```python
from build123d import *

# Parameters (mm, degrees)
SKETCH1_W                                      = 57.14999999999999
SKETCH1_H                                      = 43.17999999999999
BASE_DEPTH                                     = 57.15
POCKET_DEPTH                                   = 47.9552
LINACTHOLE_DEPTH                               = 68.44465304974146
ROLLMOTORHOLE_REACH                            = 85.656
DVIHOLE_REACH                                  = 69.445
CBORE_FOR_4_SOCKET_HEAD_CAP_SCREW1_D           = 3.2639
CBORE_FOR_4_SOCKET_HEAD_CAP_SCREW1_CBORE_D     = 6.35
CBORE_FOR_4_SOCKET_HEAD_CAP_SCREW1_CBORE_DEPTH = 2.8448
CBORE_FOR_8_SOCKET_HEAD_CAP_SCREW1_D           = 4.4958
CBORE_FOR_8_SOCKET_HEAD_CAP_SCREW1_CBORE_D     = 7.9375
CBORE_FOR_8_SOCKET_HEAD_CAP_SCREW1_CBORE_DEPTH = 4.1656
FILLET1_R                                      = 0.254


with BuildPart() as part:
    # Sketch1 → Base (new body)
    with BuildSketch(Plane(origin=(0, 0, 0), x_dir=(1, 0, 0), z_dir=(0, 1, 0))):
        Rectangle(SKETCH1_W, SKETCH1_H)
    extrude(amount=BASE_DEPTH)

    # Sketch2 → Pocket (cut)
    with BuildSketch(Plane(origin=(0, 57.15, 0), x_dir=(1, 0, 0), z_dir=(0, 1, 0))):
        Polygon((26.035000000000004, -19.05), (-26.03499999999999, -19.050000000000008), (-26.03499999999999, 19.049999999999994), (26.035000000000004, 19.050000000000004), align=None)
    extrude(amount=-POCKET_DEPTH, mode=Mode.SUBTRACT)

    # Sketch3 → LinActHole (cut, through all)
    with BuildSketch(Plane(origin=(0, 0, 0), x_dir=(-1, 0, 0), z_dir=(0, -1, 0))):
        Polygon((7.492999999999988, -7.7470000000000026), (-10.79500000000001, -7.747000000000003), (-10.79500000000001, 7.746999999999995), (7.492999999999988, 7.746999999999996), align=None)
    extrude(amount=-LINACTHOLE_DEPTH, mode=Mode.SUBTRACT)

    # Sketch4 → RollMotorHole (cut, up to next)
    with BuildSketch(Plane.ZY.offset(28.575), mode=Mode.PRIVATE) as rollmotorhole_sk1:
        Polygon((15.747999999999998, 57.15), (-4.317999999999999, 57.150000000000006), (-4.317999999999998, 47.625), (15.747999999999998, 47.625000000000014), align=None)
    rollmotorhole_tool1 = extrude(rollmotorhole_sk1.sketch, amount=-ROLLMOTORHOLE_REACH, mode=Mode.PRIVATE) & part.part
    add(rollmotorhole_tool1.solids().sort_by_distance((-28.575, 52.3875, 5.715))[0], mode=Mode.SUBTRACT)

    # Sketch5 → DviHole (cut, up to next)
    with BuildSketch(Plane.XZ, mode=Mode.PRIVATE) as dvihole_sk1:
        with BuildLine():
            Line((17.624947542752004, -13.715999999999998), (24.228947542752003, -13.716))
            Line((24.228947542752003, -13.716), (24.228947542752003, 13.716000000000003))
            Line((24.228947542752003, 13.716000000000003), (17.624947542752004, 13.716000000000005))
            ThreePointArc((17.624947542752004, 13.716000000000005), (15.828896318538174, 12.972051224213832), (15.084947542752005, 11.176000000000002))
            Line((15.084947542752005, 11.176000000000002), (15.084947542752005, -11.175999999999998))
            ThreePointArc((15.084947542752005, -11.175999999999998), (15.828896318538174, -12.972051224213828), (17.624947542752004, -13.715999999999998))
        make_face()
    dvihole_tool1 = extrude(dvihole_sk1.sketch, amount=-DVIHOLE_REACH, mode=Mode.PRIVATE) & part.part
    add(dvihole_tool1.solids().sort_by_distance((19.701649, 0, 0))[0], mode=Mode.SUBTRACT)

    # CBORE for #4 Socket Head Cap Screw1 (through all)
    with Locations(Plane(origin=(0, 0, 0), x_dir=(-1, 0, 0), z_dir=(0, -1, 0))):
        with Locations((-19.656947543, 16.256), (-19.656947543, -16.256)):
            CounterBoreHole(CBORE_FOR_4_SOCKET_HEAD_CAP_SCREW1_D / 2, CBORE_FOR_4_SOCKET_HEAD_CAP_SCREW1_CBORE_D / 2, CBORE_FOR_4_SOCKET_HEAD_CAP_SCREW1_CBORE_DEPTH)

    # CBORE for #8 Socket Head Cap Screw1 (through all)
    with Locations(Plane(origin=(0, 0, 0), x_dir=(-1, 0, 0), z_dir=(0, -1, 0))):
        with Locations((3.175, 14.605), (3.175, -14.605)):
            CounterBoreHole(CBORE_FOR_8_SOCKET_HEAD_CAP_SCREW1_D / 2, CBORE_FOR_8_SOCKET_HEAD_CAP_SCREW1_CBORE_D / 2, CBORE_FOR_8_SOCKET_HEAD_CAP_SCREW1_CBORE_DEPTH)

    # Fillet1
    # the kernel refuses this fillet: 0.254 mm, written as the material it takes off along each edge
    with BuildSketch(Plane(origin=(21.56194754300001, 2.8448, 13.716000000000006), x_dir=(1, 0, -5.46e-15), z_dir=(0, -1, 0))) as fillet1_piece_1:
        with BuildLine():
            CenterArc((0.6508256982823206, 0.25399999999999956), FILLET1_R, 138.18968510422349, 131.8103148957768)
            ThreePointArc((0.4615052761873327, 0.4233333333333256), (0.24121576475939824, 0.20026008045803986), (0, 0))
            Line((0, 0), (0.650825698282322, 0))
        make_face()
    extrude(amount=4.471864245705805, mode=Mode.SUBTRACT)
    with BuildSketch(Plane(origin=(17.751947542999993, 2.8448, 13.716000000000006), x_dir=(-0.9977003347705025, 0, -0.06777936263220105), z_dir=(0, -1, 0))) as fillet1_piece_2:
        with BuildLine():
            CenterArc((0.5964633639844708, -0.2525550871245977), FILLET1_R, 96.11431340709308, 122.7684855876463)
            Line((0.3987417282209075, -0.4119983521155698), (0.37896956464454973, -0.4279426786146676))
            ThreePointArc((0.37896956464454973, -0.4279426786146676), (0.19043822259418336, -0.21464439732501625), (-0.01658222975058737, -0.01924031331602186))
            Line((-0.01658222975058737, -0.01924031331602186), (0.00172159581085787, 0.02534158850317019))
            ThreePointArc((0.00172159581085787, 0.02534158850317019), (0.12842953857413036, 0.01673360943207212), (0.5667037799709318, 0.02525550871246005))
            Line((0.5667037799709318, 0.02525550871246005), (0.5694091966994345, 0))
        make_face()
    extrude(amount=4.278191101484826, mode=Mode.SUBTRACT)
    with BuildSketch(Plane(origin=(17.751947543000007, 2.8448, -13.715999999999996), x_dir=(-0.9977003347705027, 0, 0.06777936263219668), z_dir=(0, -1, 0))) as fillet1_piece_3:
        with BuildLine():
            CenterArc((0.5964633639844823, 0.25255508712459757), FILLET1_R, 141.1172010052604, 122.76848558764627)
            Line((0.3987417282209198, 0.4119983521155705), (0.37896956464456205, 0.4279426786146684))
            ThreePointArc((0.37896956464456205, 0.4279426786146684), (0.19043822259419124, 0.21464439732501767), (-0.01658222975058728, 0.01924031331602193))
            Line((-0.01658222975058728, 0.01924031331602193), (0.00172159581085776, -0.02534158850317019))
            ThreePointArc((0.00172159581085776, -0.02534158850317019), (0.12842953857414433, -0.01673360943206995), (0.5667037799709422, -0.02525550871246003))
            Line((0.5667037799709422, -0.02525550871246003), (0.5694091966994449, 0))
        make_face()
    extrude(amount=4.278191101484849, mode=Mode.SUBTRACT)
    with BuildSketch(Plane(origin=(21.561947542999995, 2.8448, -13.715999999999996), x_dir=(1, 0, -5.46e-15), z_dir=(0, -1, 0))) as fillet1_piece_4:
        with BuildLine():
            CenterArc((0.6508256982823268, -0.25399999999999956), FILLET1_R, 90.0000000000003, 131.81031489577913)
            ThreePointArc((0.46150527618734805, -0.42333333333333484), (0.2412157647594075, -0.20026008045804258), (0, 0))
            Line((0, 0), (0.6508256982823255, 0))
        make_face()
    extrude(amount=4.471864245705815, mode=Mode.SUBTRACT)


solid = part.part
```
Design review of the part built by this model. Coordinates are the model's own, in mm. A direction names the side the tool comes from. Round coordinates to 2 decimals unless told otherwise and drop trailing zeros. Write each loop counter-clockwise with the first axis right and the second up, starting at its lowest first coordinate (ties: lowest second). Pieces come first, ordered by that corner, then holes. Notation, with made-up numbers: (3.25, 19.25) -> (16.25, 19.25) arc R8 cw to (16.25, 30.25) -> close; hole circle Ø7 at (39.25, -40). An arc over 180 degrees is marked (long way). Answer in a Markdown table with one row per item.
Q1. Draft analysis for pull direction Z (two halves, no side actions). For faces 5 (the face through (-11, 9.195, 0)), 6 (the face through (0, 0, -10)), state which applies: +Z half, -Z half, draft (parallel to the pull), parting line (faces both ways), or undercut.
The answers:
| item | result |
|---|---|
| face 5 | undercut |
| face 6 | draft |
Q2. Take a section at B-B, the plane x = 8. State the section outline as (y, z) points, then the cut area to 3 significant figures.
The answers:
| item | result |
|---|---|
| outline | (0, -21.59) -> (57.15, -21.59) -> (57.15, -19.05) -> (9.19, -19.05) -> (9.19, -7.75) -> (0, -7.75) -> close; (0, 7.75) -> (9.19, 7.75) -> (9.19, 19.05) -> (57.15, 19.05) -> (57.15, 21.59) -> (0, 21.59) -> close |
| area | 498 mm² |
Q3. Take a section at C-C, the plane y = 44. State the section outline as (x, z) points (3 decimals).
The answers:
| item | result |
|---|---|
| outline | (-28.575, -21.59) -> (28.575, -21.59) -> (28.575, 21.59) -> (-28.575, 21.59) -> close; hole (-26.035, -19.05) -> (26.035, -19.05) -> (26.035, 19.05) -> (-26.035, 19.05) -> close |
Q4. Clearance check with flat-ended pins moving along their axes: pin 1 Ø7 at (x, z) = (-3.175, -14.605) entering from -Y; pin 2 Ø6 at (x, z) = (-3.175, 14.605) entering from +Y; pin 3 Ø0.8 at (x, z) = (-27.5, 5.5) entering from +Y (3 decimals). State where each tip first meets the part, or that it passes through.
The answers:
| item | result |
|---|---|
| pin 1 | y = 4.17 |
| pin 2 | y = 9.19 |
| pin 3 | y = 47.625 |
Q5. For faces 1 (the face through (-5, 4.166, -13)), 2 (the face through (-27, 52, -4.318)), 3 (the face through (0, 34, -19.05)), 4 (the face through (15.849, 4.533, 12.992)), list the 3-axis set-ups (+Z, -Z, +X, -X, +Y, -Y) from which the entire face can be reached by the end or side of a thin tool; tool diameter is ignored.
The answers:
| item | result |
|---|---|
| face 1 | -Y |
| face 2 | -X, +Y |
| face 3 | +Y |
| face 4 | +Y, -Y |
Q6. Take a section at A-A, the plane z = -0.5. State the section outline as (x, y) points (3 decimals).
The answers:
| item | result |
|---|---|
| outline | (-28.575, 0) -> (-7.493, 0) -> (-7.493, 9.195) -> (-26.035, 9.195) -> (-26.035, 47.625) -> (-28.575, 47.625) -> close; (10.795, 0) -> (15.085, 0) -> (15.085, 9.195) -> (10.795, 9.195) -> close; (24.229, 0) -> (28.575, 0) -> (28.575, 57.15) -> (26.035, 57.15) -> (26.035, 9.195) -> (24.229, 9.195) -> close |
Q7. Take a section at D-D, the plane y = 5.5. State the section outline as (x, z) points (3 decimals), then the cut area to 3 significant figures.
The answers:
| item | result |
|---|---|
| outline | (-28.575, -21.59) -> (28.575, -21.59) -> (28.575, 21.59) -> (-28.575, 21.59) -> close; hole (-7.493, -7.747) -> (10.795, -7.747) -> (10.795, 7.747) -> (-7.493, 7.747) -> close; hole circle Ø4.496 at (-3.175, -14.605); hole circle Ø4.496 at (-3.175, 14.605); hole (15.085, -11.176) arc R2.54 ccw to (17.625, -13.716) -> (24.229, -13.716) -> (24.229, 13.716) -> (17.625, 13.716) arc R2.54 ccw to (15.085, 11.176) -> close; hole circle Ø3.264 at (19.657, -16.256); hole circle Ø3.264 at (19.657, 16.256) |
| area | 1,890 mm² |
Q8. To check wall thickness, follow L1, parallel to X at y = 7, z = 2.5 (3 decimals); L2, parallel to X at y = 25.5, z = -5.5 (3 decimals); L3, parallel to Z at x = -1.5, y = 28. State the ranges of each line that lie inside material, in increasing order. Write a range as [from, to].
The answers:
| item | result |
|---|---|
| L1 | [-28.575, -7.493], [10.795, 15.085], [24.229, 28.575] |
| L2 | [-28.575, -26.035], [26.035, 28.575] |
| L3 | [-21.59, -19.05], [19.05, 21.59] |
